from build123d import *

# Parameters (mm, degrees)
F1_DEPTH = 19.05
F3_DEPTH = 19.05


with BuildPart() as f1:
    # F0 (on Right) → F1 (new body)
    with BuildSketch(Plane.YZ):
        Polygon((0, 60.502801), (0, 0), (76.2, 0), (76.2, 38.1), (50.901599, 60.502801), align=None)
    extrude(amount=F1_DEPTH)

    # F2 (on face) → F3 (join)
    with BuildSketch(Plane.YZ.offset(19.05)):
        Polygon((0, 0), (38.1, 0), (0, 60.502801), align=None)
    extrude(amount=F3_DEPTH)


solid = f1.part
The model under review builds one solid part; all positions refer to its coordinate system, in mm. A direction names the side the tool comes from. Coordinates: 2 decimals unless noted, no trailing zeros. Write each loop counter-clockwise with the first axis right and the second up, starting at its lowest first coordinate (ties: lowest second). Pieces come first, ordered by that corner, then holes. Notation, with made-up numbers: (25, -13) - (81, -13) arc R13 ccw to (81, -1) - close; hole circle Ø5 at (-16, -21). An arc over 180 degrees is marked (long way). Answer as CSV lines item,"result".
(1) We need section C-C (z = 22). Give the boundary of the cut face in (x, y).
Data:
outline,"(0, 0) - (38.1, 0) - (38.1, 24.25) - (19.05, 24.25) - (19.05, 76.2) - (0, 76.2) - close"
(2) Tool access review of faces 1 (the flat face through (19, 0, 31)), 2 (the flat face through (28.442, 19.317, 29.828)): name each direction out of +Z, -Z, +X, -X, +Y, -Y from which nothing blocks a thin tool from reaching the whole face with its end or side.
Data:
face 1,"+Z, -Z, +X, -X, -Y"
face 2,"+Z, +X, +Y"
(3) Clearance check with flat-ended pins moving along their axes: pin 1 Ø10 at (y, z) = (65, 14) entering from +X; pin 2 Ø10 at (x, y) = (24.5, 27) entering from +Z. State where each tip first meets the part, or that it passes through.
Data:
pin 1,"stops at x = 19.05"
pin 2,"stops at z = 25.57"
(4) We need section A-A (x = 29). Give the boundary of the cut face in (y, z), plus the area to 3 significant figures.
Data:
outline,"(0, 0) - (38.1, 0) - (0, 60.5) - close"
area,"1,150 mm2"
(5) We need section D-D (y = 9.5). Give the boundary of the cut face in (x, z).
Data:
outline,"(0, 0) - (38.1, 0) - (38.1, 45.42) - (19.05, 45.42) - (19.05, 60.5) - (0, 60.5) - close"
(6) For line 1 along X through (y, z) = (46, 48.5); line 2 along Y through (x, z) = (33, 34.5); line 3 along Z through (x, y) = (35, 16.5), list the stretches that pass through material, from the lowest coordinate up. Write a range as [from, to].
Data:
line 1,"x = [0, 19.05]"
line 2,"y = [0, 16.37]"
line 3,"z = [0, 34.3]"
(7) We need section B-B (y = 46). Give the boundary of the cut face in (x, z).
Data:
outline,"(0, 0) - (19.05, 0) - (19.05, 60.5) - (0, 60.5) - close"
